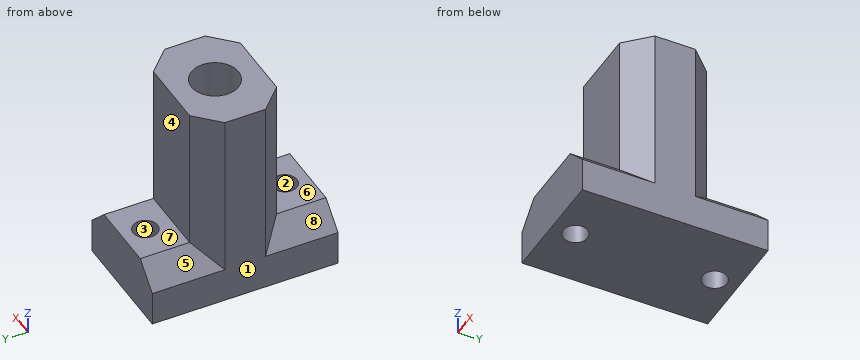
from build123d import *

# Parameters (mm, degrees)
F1_DEPTH = 10
F3_DEPTH = 25
F4_SIZE  = 4
F5_R     = 2.1
F6_DEPTH = 10.001
F7_R     = 4.05
F8_DEPTH = 25
F9_SIZE  = 4


with BuildPart() as f1:
    # F0 (on Top) → F1 (new body)
    with BuildSketch(Plane.XY):
        Polygon((-10, 16), (-10, 0), (-10, -16), (0, -16), (10, -16), (10, 0), (10, 16), (0, 16), align=None)
    extrude(amount=F1_DEPTH)

    # F2 (on face) → F3 (join)
    with BuildSketch(Plane.XY.offset(10)):
        Polygon((10, 7.5), (0, 7.5), (-10, 7.5), (-10, -7.5), (0, -7.5), (10, -7.5), (10, 0), align=None)
    extrude(amount=F3_DEPTH)

    # F4
    f4_edges = [f1.edges().sort_by_distance(p)[0] for p in [
        (-10, -7.5, 22.5),
        (10, -7.5, 22.5),
        (10, 7.5, 22.5),
        (-10, 7.5, 22.5),
    ]]
    chamfer(f4_edges, length=F4_SIZE)

    # F5 (on face) → F6 (cut, through all)
    with BuildSketch(Plane.XY.offset(10)):
        with Locations((0, 12)):
            Circle(F5_R)
        with Locations((0, -12)):
            Circle(F5_R)
    extrude(amount=-F6_DEPTH, mode=Mode.SUBTRACT)

    # F7 (on face) → F8 (cut)
    with BuildSketch(Plane.XY.offset(35)):
        Circle(F7_R)
    extrude(amount=-F8_DEPTH, mode=Mode.SUBTRACT)

    # F9
    f9_edges = [f1.edges().sort_by_distance(p)[0] for p in [
        (-10, 9.75, 10),
        (-10, -9.75, 10),
        (10, -9.75, 10),
        (10, 9.75, 10),
    ]]
    chamfer(f9_edges, length=F9_SIZE)


solid = f1.part
The listing builds one solid part. Answer for the finished solid, in the listing's coordinates (mm). Face numbers are marked on the shaded views. A direction names the side the tool comes from. Round coordinates to 2 decimals unless told otherwise and drop trailing zeros. Write each loop counter-clockwise with the first axis right and the second up, starting at its lowest first coordinate (ties: lowest second). Pieces come first, ordered by that corner, then holes. Notation, with made-up numbers: (-23.5, -2.75) - (10.5, -2.75) arc R27 ccw to (10.5, 18.25) - close; hole circle Ø5 at (76.5, 57.5). An arc over 180 degrees is marked (long way). Use one line per item in the form item = value. Start each with the question number.
Item 1: A tool of negligible diameter and unlimited length cuts with its end or side. For the marked faces 5, 6, 7 and 8, from which of +Z, -Z, +X, -X, +Y, -Y can it reach the whole face along a straight path? Write none if from no direction.
Item 2: A cutting plane is placed at D-D (x = -5.5). Write down the section's boundary in (y, z), plus the area to 3 significant figures.
Item 3: A cutting plane is placed at A-A (x = 0). Write down the section's boundary in (y, z), plus the area to 4 significant figures.
Item 4: Find the intervals of material crossed by line 1 (Y direction, x = 0, z = 7); line 2 (Y direction, x = 0, z = 20); line 3 (Z direction, x = -1, y = 1.5), in increasing order. Write a range as [from, to].
Item 5: Determine the mould class of the marked faces 1, 2, 3 and 4 for opening direction Y: +Y half, -Y half, draft (parallel to the pull), parting line (faces both ways), or undercut.
Item 6: Flat-ended cylindrical pins translate along their axes: pin 1 Ø5 at (x, y) = (4.5, 9.5) entering from -Z; pin 2 Ø6.5 at (x, y) = (0, -12) entering from +Z; pin 3 Ø3.5 at (x, z) = (-2, 27.5) entering from +Y; pin 4 Ø2 at (x, z) = (2.5, 24.5) entering from -Y. Find the tip coordinate at first contact, or state that the pin passes through.
Item 7: A cutting plane is placed at C-C (z = 32.5). Write down the section's boundary in (x, y), plus the area to 3 significant figures.
Item 8: A cutting plane is placed at B-B (y = 12). Write down the section's boundary in (x, z), plus the area to 3 significant figures.
The answers:
q1.face_5 = +Z, -X, +Y
q1.face_6 = +Z, +X, -X, -Y
q1.face_7 = +Z, +X, -X, +Y
q1.face_8 = +Z, -X, -Y
q2.outline = (-16, 0) - (16, 0) - (16, 10) - (7.5, 10) - (7.5, 35) - (-7.5, 35) - (-7.5, 10) - (-16, 10) - close
q2.area = 695 mm^2
q3.outline = (-16, 0) - (-14.1, 0) - (-14.1, 10) - (-16, 10) - close; (-9.9, 0) - (9.9, 0) - (9.9, 10) - (7.5, 10) - (7.5, 35) - (4.05, 35) - (4.05, 10) - (-4.05, 10) - (-4.05, 35) - (-7.5, 35) - (-7.5, 10) - (-9.9, 10) - close; (14.1, 0) - (16, 0) - (16, 10) - (14.1, 10) - close
q3.area = 408.5 mm^2
q4.line_1 = [-16, -14.1], [-9.9, 9.9], [14.1, 16]
q4.line_2 = [-7.5, -4.05], [4.05, 7.5]
q4.line_3 = [0, 10]
q5.face_1 = draft
q5.face_2 = undercut
q5.face_3 = undercut
q5.face_4 = +Y half
q6.pin_1 = 0
q6.pin_2 = 10
q6.pin_3 = 7.5
q6.pin_4 = -7.5
q7.outline = (-10, -3.5) - (-6, -7.5) - (6, -7.5) - (10, -3.5) - (10, 3.5) - (6, 7.5) - (-6, 7.5) - (-10, 3.5) - close; hole circle Ø8.1 at (0, 0)
q7.area = 216 mm^2
q8.outline = (-10, 0) - (-2.1, 0) - (-2.1, 10) - (-6, 10) - (-10, 6) - close; (2.1, 0) - (10, 0) - (10, 6) - (6, 10) - (2.1, 10) - close
q8.area = 142 mm^2
